from build123d import *
from build123d.topology import SkipClean

# Parameters (mm, degrees)
SKETCH1_R           = 10
SKETCH1_R_2         = 1.5
SKETCH1_R_3         = 0.825
BOSS_EXTRUDE1_DEPTH = 3.5
BOSS_EXTRUDE2_START = 2
SKETCH2_R           = 4.5
SKETCH2_R_2         = 1.5
BOSS_EXTRUDE2_DEPTH = 2
SKETCH3_R           = 3
CUT_EXTRUDE1_DEPTH  = 3.5
CHAMFER1_SIZE       = 0.5


with BuildPart() as part:
    # Sketch1 → Boss-Extrude1 (new body)
    with BuildSketch(Plane(origin=(0, 0, 0), x_dir=(1, 0, 0), z_dir=(0, 1, 0))):
        with Locations(Location((0, 0, 0), (0, 0, 270))):
            Circle(SKETCH1_R)
        with Locations(Location((0, 0, 0), (0, 0, 270))):
            Circle(SKETCH1_R_2, mode=Mode.SUBTRACT)
        with Locations(Location((0, 7, 0), (0, 0, 270))):
            Circle(SKETCH1_R_3, mode=Mode.SUBTRACT)
        with Locations(Location((7, 0, 0), (0, 0, 270))):
            Circle(SKETCH1_R_3, mode=Mode.SUBTRACT)
        with Locations(Location((0, -7, 0), (0, 0, 270))):
            Circle(SKETCH1_R_3, mode=Mode.SUBTRACT)
        with Locations(Location((-7, 0, 0), (0, 0, 270))):
            Circle(SKETCH1_R_3, mode=Mode.SUBTRACT)
    extrude(amount=BOSS_EXTRUDE1_DEPTH)

    # Sketch2 → Boss-Extrude2 (add)
    with SkipClean():  # the faces are left unmerged after this step: merging them gives an invalid solid
        with BuildSketch(Plane.XZ.offset(BOSS_EXTRUDE2_START)):
            with Locations(Location((0, 0, 0), (0, 0, 90))):
                Circle(SKETCH2_R)
            with Locations(Location((0, 0, 0), (0, 0, 270))):
                Circle(SKETCH2_R_2, mode=Mode.SUBTRACT)
        extrude(amount=-BOSS_EXTRUDE2_DEPTH)

    # Sketch3 → Cut-Extrude1 (cut)
    with BuildSketch(Plane.XZ.offset(2)):
        with Locations(Location((0, 0, 0), (0, 0, 270))):
            Circle(SKETCH3_R)
    extrude(amount=-CUT_EXTRUDE1_DEPTH, mode=Mode.SUBTRACT)

    # Chamfer1
    chamfer1_edges = [part.edges().sort_by_distance(p)[0] for p in [
        (0, -2, 3),
    ]]
    chamfer(chamfer1_edges, length=CHAMFER1_SIZE)


solid = part.part
Verification items for the finished model (mm, model axes). A direction names the side the tool comes from. Give positions to 0.01 mm unless a question says otherwise; leave off trailing zeros. Loops run counter-clockwise (first coordinate to the right, second up) from the corner with the lowest first, then second, coordinate; pieces in that order, holes last.
1. Cross-section at C-C on z = 7.5. Record the cut outline in (x, y).
Derived:
outline: (-6.61, 0) - (-0.66, 0) - (-0.66, 3.5) - (-6.61, 3.5) - close; (0.66, 0) - (6.61, 0) - (6.61, 3.5) - (0.66, 3.5) - close
2. Release check for a two-part mould opening along X. For faces 1 (the flat face through (-2, 3.5, 0)), 2 (the cylindrical face through (-9.76, 1.73, -2.17)), 3 (the flat face through (-1.3, 1.5, -1.3)) record: +X half, -X half, draft (parallel to the pull), parting line (faces both ways), or undercut.
Derived:
face 1: draft
face 2: parting line
face 3: undercut
3. Cross-section at A-A on x = 0. Record the cut outline in (y, z) (3 decimals), and give its area (3 significant figures).
Derived:
outline: (-2, -4.5) - (0, -4.5) - (0, -6.175) - (3.5, -6.175) - (3.5, -1.5) - (1.5, -1.5) - (1.5, -3) - (-1.5, -3) - (-2, -3.5) - close; (-2, 3.5) - (-1.5, 3) - (1.5, 3) - (1.5, 1.5) - (3.5, 1.5) - (3.5, 6.175) - (0, 6.175) - (0, 4.5) - (-2, 4.5) - close; (0, -10) - (3.5, -10) - (3.5, -7.825) - (0, -7.825) - close; (0, 7.825) - (3.5, 7.825) - (3.5, 10) - (0, 10) - close
area: 49.2 mm2
4. Cross-section at B-B on y = 0.4. Record the cut outline in (x, z) (3 decimals).
Derived:
outline: circle Ø20 at (0, 0); hole circle Ø1.65 at (-7, 0); hole circle Ø6 at (0, 0); hole circle Ø1.65 at (0, -7); hole circle Ø1.65 at (0, 7); hole circle Ø1.65 at (7, 0)
5. Material ranges on probe 1 along X at (y, z) = (1.7, 0) (3 decimals); probe 2 along X at (y, z) = (-0.6, 0); probe 3 along Y at (x, z) = (-5, 2.25), recorded low to high.
Derived:
probe 1: x = -10 to -7.825, -6.175 to -1.5, 1.5 to 6.175, 7.825 to 10
probe 2: x = -4.5 to -3, 3 to 4.5
probe 3: y = 0 to 3.5
6. Go/stop test with flat-tipped pins: P1, Ø2.5, axis at x = 0, z = 0, coming from the +Y side; P2, Ø2, axis at x = -7, z = 0, coming from the -Y side; P3, Ø10, axis at x = 1.5, z = -7.5, coming from the -Y side; P4, Ø3, axis at x = -0.5, z = 0.5, coming from the -Y side. Record where each tip stops, or that it passes through.
Derived:
P1: passes through
P2: stops at y = 0
P3: stops at y = -2
P4: stops at y = 1.5
7. Tool access check on faces 4 (the cylindrical face through (-0.32, 1.73, 7.76)), 5 (the cylindrical face through (0.9, -0.02, -2.86)). Record the directions out of +Z, -Z, +X, -X, +Y, -Y that give a thin tool (end or side, any length) a straight path to the whole face; none if there is none.
Derived:
face 4: +Y, -Y
face 5: -Y
8. Cross-section at D-D on z = 0. Record the cut outline in (x, y) (3 decimals).
Derived:
outline: (-10, 0) - (-7.825, 0) - (-7.825, 3.5) - (-10, 3.5) - close; (-6.175, 0) - (-4.5, 0) - (-4.5, -2) - (-3.5, -2) - (-3, -1.5) - (-3, 1.5) - (-1.5, 1.5) - (-1.5, 3.5) - (-6.175, 3.5) - close; (1.5, 1.5) - (3, 1.5) - (3, -1.5) - (3.5, -2) - (4.5, -2) - (4.5, 0) - (6.175, 0) - (6.175, 3.5) - (1.5, 3.5) - close; (7.825, 0) - (10, 0) - (10, 3.5) - (7.825, 3.5) - close
